Build history of the part. All positions in model axes, mm. Face numbers are marked on the shaded views. A direction names the side the tool comes from. Give positions to 0.01 mm unless a question says otherwise; leave off trailing zeros. Order: outer loops, then holes, each group sorted by start corner. A loop starts at its lowest first (then second) coordinate and runs counter-clockwise, first axis right, second up. Notation, with made-up numbers: M 76,56.5 L 84,56.5 A13 cw 84,65.5 Z; hole C -22,-35.5 d6. An arc over 180 degrees is marked long. One line per item, written item: value.
from build123d import *

# Parameters (mm, degrees)
F0_W     = 69.926764816
F0_H     = 71.7419460416
F1_DEPTH = 25.4
F3_R     = 23.8517275111
F4_DEPTH = 38.1
F5_R     = 12.5762061787
F6_DEPTH = 63.501


with BuildPart() as f1:
    # F0 (on Front) → F1 (new body)
    with BuildSketch(Plane.XZ):
        with Locations((3.1551141292, 0.7052309811)):
            Rectangle(F0_W, F0_H)
    extrude(amount=F1_DEPTH)

    # F3 (on face) → F4 (join)
    with BuildSketch(Plane.XZ.offset(25.4)):
        with Locations((4.5831017196, 0)):
            Circle(F3_R)
    extrude(amount=F4_DEPTH)

    # F5 (on face) → F6 (cut, through all)
    with BuildSketch(Plane.XZ.offset(63.5)):
        with Locations((4.8407912254, 0)):
            Circle(F5_R)
    extrude(amount=-F6_DEPTH, mode=Mode.SUBTRACT)


solid = f1.part
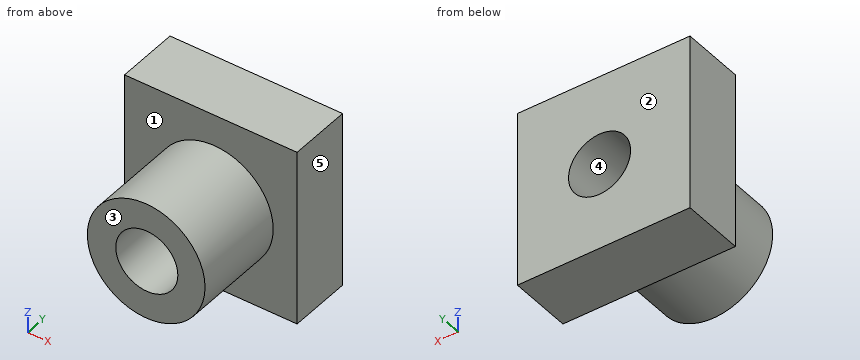
1) Saw through at D-D, the plane x = 22. Write the cut outline in (y, z).
Check values:
outline: M -63.5,-16.3 L -25.4,-16.3 L -25.4,-35.17 L 0,-35.17 L 0,36.58 L -25.4,36.58 L -25.4,16.3 L -63.5,16.3 Z
2) Saw through at B-B, the plane x = 5.5. Write the cut outline in (y, z).
Check values:
outline: M -63.5,-23.83 L -25.4,-23.83 L -25.4,-35.17 L 0,-35.17 L 0,-12.56 L -63.5,-12.56 Z; M -63.5,12.56 L 0,12.56 L 0,36.58 L -25.4,36.58 L -25.4,23.83 L -63.5,23.83 Z
3) Pin check, flat tips, straight feed: pin 1 (4 mm diameter, centred on y = -30, z = -14, fed in from -X); pin 2 (8 mm diameter, centred on x = -24.5, y = -32.5, fed in from +Z); pin 3 (2 mm diameter, centred on y = -27, z = -8.5, fed in from -X). Stop position of each tip, or through.
Check values:
pin 1: x = -16.03
pin 2: through
pin 3: x = -18.06
4) Saw through at A-A, the plane z = 0. Write the cut outline in (x, y), then the cut area to 3 significant figures.
Check values:
outline: M -31.81,-25.4 L -19.27,-25.4 L -19.27,-63.5 L -7.74,-63.5 L -7.74,0 L -31.81,0 Z; M 17.42,-63.5 L 28.43,-63.5 L 28.43,-25.4 L 38.12,-25.4 L 38.12,0 L 17.42,0 Z
area: 2,000 mm^2
5) Saw through at C-C, the plane y = -13. Write the cut outline in (x, z), then the cut area to 3 significant figures.
Check values:
outline: M -31.81,-35.17 L 38.12,-35.17 L 38.12,36.58 L -31.81,36.58 Z; hole C 4.84,0 d25.15
area: 4,520 mm^2
6) Tool access for the marked faces 1 and 2: list every direction of +Z, -Z, +X, -X, +Y, -Y with a clear straight run to the whole face (end or side of a thin tool).
Check values:
face 1: -Y
face 2: +Z, -Z, +X, -X, +Y
7) Drill centre lines: probe 1 along Y at (x, z) = (-17, -15); probe 2 along Z at (x, y) = (16, -37.5); probe 3 along Z at (x, y) = (4, -52). Where is each one in solid material? Low to high. Write a range as from..to.
Check values:
probe 1: -25.4..0
probe 2: -20.94..-5.8, 5.8..20.94
probe 3: -23.84..-12.55, 12.55..23.84
8) Mould opens along X. For the marked faces 3, 4 and 5 say: released by +X, released by -X, zero draft, split by the parting line, or undercut.
Check values:
face 3: zero draft
face 4: undercut
face 5: released by +X
